from build123d import *

# Parameters (mm, degrees)
SKETCH1_W                                           = 150
SKETCH1_H                                           = 150
BOSS_EXTRUDE1_DEPTH                                 = 10
SKETCH2_R                                           = 45
SKETCH2_W                                           = 41
SKETCH2_H                                           = 21
BOSS_EXTRUDE2_DEPTH                                 = 35
SKETCH3_W                                           = 57
SKETCH3_H                                           = 21
CUT_EXTRUDE1_DEPTH                                  = 13
SKETCH5_W                                           = 57
SKETCH5_H                                           = 21
CUT_EXTRUDE3_DEPTH                                  = 29
RIB5_REACH                                          = 117.217
SKETCH6_WALL_W                                      = 276.297796834
SKETCH6_WALL_H                                      = 10
CIRPATTERN1_COUNT                                   = 4
CSK_FOR_M5_COUNTERSUNK_FLAT_HEAD_SCREW1_D           = 5.5
CSK_FOR_M5_COUNTERSUNK_FLAT_HEAD_SCREW1_CSINK_D     = 10.4
CSK_FOR_M5_COUNTERSUNK_FLAT_HEAD_SCREW1_CSINK_ANGLE = 90
SKETCH12_R                                          = 2.5
CUT_EXTRUDE4_DEPTH                                  = 10
CUT_EXTRUDE5_DEPTH                                  = 144.449259322
CUT_EXTRUDE5_DEPTH_BACK                             = 144.449259322
SKETCH13_W                                          = 5.5
SKETCH13_H                                          = 4


with BuildPart() as part:
    # Sketch1 → Boss-Extrude1 (new body)
    with BuildSketch(Plane(origin=(0, 0, 0), x_dir=(1, 0, 0), z_dir=(0, 1, 0))):
        Rectangle(SKETCH1_W, SKETCH1_H)
    extrude(amount=BOSS_EXTRUDE1_DEPTH)

    # Sketch2 → Boss-Extrude2 (add)
    with BuildSketch(Plane(origin=(0, 10, 0), x_dir=(1, 0, 0), z_dir=(0, 1, 0))):
        with Locations(Location((0, 0, 0), (0, 0, 270))):
            Circle(SKETCH2_R)
        with Locations((-10.2, 0)):
            Rectangle(SKETCH2_W, SKETCH2_H, mode=Mode.SUBTRACT)
    extrude(amount=BOSS_EXTRUDE2_DEPTH)

    # Sketch3 → Cut-Extrude1 (cut)
    with BuildSketch(Plane(origin=(0, 45, 0), x_dir=(1, 0, 0), z_dir=(0, 1, 0))):
        with Locations((-10.2, 0)):
            Rectangle(SKETCH3_W, SKETCH3_H)
    extrude(amount=-CUT_EXTRUDE1_DEPTH, mode=Mode.SUBTRACT)

    # Sketch5 → Cut-Extrude3 (cut)
    with BuildSketch(Plane.XZ):
        with Locations((-10.2, 0)):
            Rectangle(SKETCH5_W, SKETCH5_H)
    extrude(amount=-CUT_EXTRUDE3_DEPTH, mode=Mode.SUBTRACT)

    # Sketch6 wall → Rib5 (add, up to next)
    with BuildSketch(Plane(origin=(0, 26, -60), x_dir=(0, -0.72953720414, -0.683941128881), z_dir=(0, 0.683941128881, -0.72953720414)), mode=Mode.PRIVATE) as rib5_sk1:
        Rectangle(SKETCH6_WALL_W, SKETCH6_WALL_H)
    rib5_tool1 = extrude(rib5_sk1.sketch, amount=-RIB5_REACH, mode=Mode.PRIVATE) - part.part
    rib5 = rib5_tool1.solids().sort_by_distance((0, 26, -60))[0]
    add(rib5)

    # CirPattern1: Rib5 ×4 about axis
    cirpattern1_axis = Axis((0, 0, 0), (0, 1, 0))
    for i in range(1, CIRPATTERN1_COUNT):
        add(rib5.rotate(cirpattern1_axis, i * 360 / CIRPATTERN1_COUNT))

    # CSK for M5 Countersunk Flat Head Screw1 (through all)
    with Locations(Plane(origin=(0, 10, 0), x_dir=(1, 0, 0), z_dir=(0, 1, 0))):
        with Locations((55, -55), (-55, -55), (-55, 55), (55, 55)):
            CounterSinkHole(CSK_FOR_M5_COUNTERSUNK_FLAT_HEAD_SCREW1_D / 2, CSK_FOR_M5_COUNTERSUNK_FLAT_HEAD_SCREW1_CSINK_D / 2, counter_sink_angle=CSK_FOR_M5_COUNTERSUNK_FLAT_HEAD_SCREW1_CSINK_ANGLE)

    # Sketch12 → Cut-Extrude4 (cut)
    with BuildSketch(Plane(origin=(0, 32, 0), x_dir=(1, 0, 0), z_dir=(0, 1, 0))):
        with Locations(Location((-34.5, 5.25, 0), (0, 0, 270))):
            Circle(SKETCH12_R)
        with Locations(Location((-34.5, -4.75, 0), (0, 0, 270))):
            Circle(SKETCH12_R)
        with Locations(Location((14.5, 5.25, 0), (0, 0, 270))):
            Circle(SKETCH12_R)
        with Locations(Location((14.5, -5, 0), (0, 0, 270))):
            Circle(SKETCH12_R)
    extrude(amount=-CUT_EXTRUDE4_DEPTH, mode=Mode.SUBTRACT)

    # Sketch13 → Cut-Extrude5 (cut, two sides: drawn at the far end of the back side and taken through both)
    with BuildSketch(Plane(origin=(-38.7, 0, 0), x_dir=(0, 0, -1), z_dir=(1, 0, 0)).offset(-CUT_EXTRUDE5_DEPTH_BACK)):
        with Locations((0, 2)):
            Rectangle(SKETCH13_W, SKETCH13_H)
    extrude(amount=CUT_EXTRUDE5_DEPTH + CUT_EXTRUDE5_DEPTH_BACK, mode=Mode.SUBTRACT)


solid = part.part
Geometry check sheet. Reference: the model listing, model coordinates, mm. A direction names the side the tool comes from. Round coordinates to 2 decimals unless told otherwise and drop trailing zeros. Order: outer loops, then holes, each group sorted by start corner. A loop starts at its lowest first (then second) coordinate and runs counter-clockwise, first axis right, second up. Notation, with made-up numbers: M 67.5,-3 L 125.5,-3 A20 ccw 125.5,1 Z; hole C -6,-11.5 d4. An arc over 180 degrees is marked long. Answer in a Markdown table with one row per item. Add a question column.
Item 1: Draft check along X on faces 6 (the face through (-52.973, 3.722, -56.859)), 7 (the face through (5, 21, 53)), 8 (the face through (-35, 29, 0)), 9 (the face through (-48, 10, 47)). Enter one of: released by +X, released by -X, zero draft, split by the parting line, or undercut.
Item 2: Depth check by flat-ended pin: pin 1 Ø6.5 at (x, z) = (14.5, 5) entering from +Y; pin 2 Ø0.9 at (y, z) = (31, 4) entering from -X; pin 3 Ø9 at (y, z) = (19, -53) entering from +X. Enter the tip coordinate at first touch or a pass-through.
Item 3: Sectioned sample at D-D, the plane x = 55. Enter the section's corners in (y, z), plus the area to 3 significant figures.
Item 4: Sectioned sample at A-A, the plane x = 0. Enter the section's corners in (y, z), plus the area to 4 significant figures.
Item 5: Sectioned sample at B-B, the plane z = 0. Enter the section's corners in (x, y), plus the area to 3 significant figures.
Item 6: Set-up check for faces 1 (the face through (-17.235, 27.255, 41.569)), 2 (the face through (-5, 21, 53)), 3 (the face through (46, 4, 0)), 4 (the face through (53, 21, -5)), 5 (the face through (-1, 5, 75)): record each of +Z, -Z, +X, -X, +Y, -Y from which the full face is reachable in a straight line by a thin tool's end or side.
Item 7: Material ranges on L1, parallel to Z at x = -55, y = 6; L2, parallel to Z at x = 55, y = 2; L3, parallel to Z at x = -32, y = 9.5, recorded low to high. Write a range as [from, to].
Item 8: Sectioned sample at C-C, the plane y = 14. Enter the section's corners in (x, z).
Filled in:
| question | item | result |
|---|---|---|
| 1 | face 6 | undercut |
| 1 | face 7 | released by +X |
| 1 | face 8 | undercut |
| 1 | face 9 | zero draft |
| 2 | pin 1 | stops at y = 32 |
| 2 | pin 2 | stops at x = -55.73 |
| 2 | pin 3 | stops at x = 5 |
| 3 | outline | M 0,-75 L 10,-75 L 10,-60.2 L 7.55,-57.75 L 0,-57.75 Z; M 0,-52.25 L 7.55,-52.25 L 10,-49.8 L 10,-5 L 31.33,-5 L 31.33,5 L 10,5 L 10,49.8 L 7.55,52.25 L 0,52.25 L 0,2.75 L 4,2.75 L 4,-2.75 L 0,-2.75 Z; M 0,57.75 L 7.55,57.75 L 10,60.2 L 10,75 L 0,75 Z |
| 3 | area | 1,570 mm² |
| 4 | outline | M 0,-75 L 10,-75 L 42,-45 L 45,-45 L 45,-10.5 L 0,-10.5 Z; M 0,10.5 L 45,10.5 L 45,45 L 42,45 L 10,75 L 0,75 Z |
| 4 | area | 4,665 mm² |
| 5 | outline | M -75,4 L -38.7,4 L -38.7,29 L -30.7,29 L -30.7,32 L -38.7,32 L -38.7,45 L -45,45 L -45,42 L -75,10 Z; M 10.3,29 L 18.3,29 L 18.3,4 L 75,4 L 75,10 L 45,42 L 45,45 L 18.3,45 L 18.3,32 L 10.3,32 Z |
| 5 | area | 2,720 mm² |
| 6 | face 1 | +Y |
| 6 | face 2 | +Z, -X, +Y |
| 6 | face 3 | +X, -X, -Y |
| 6 | face 4 | -Z, +X, +Y |
| 6 | face 5 | +Z, +X, -X, +Y, -Y |
| 7 | L1 | z = [-75, -57.75], [-52.25, 52.25], [57.75, 75] |
| 7 | L2 | z = [-75, -57.75], [-52.25, -2.75], [2.75, 52.25], [57.75, 75] |
| 7 | L3 | z = [-75, -10.5], [10.5, 75] |
| 8 | outline | M -71.25,-5 L -44.72,-5 A45 ccw -5,-44.72 L -5,-71.25 L 5,-71.25 L 5,-44.72 A45 ccw 44.72,-5 L 71.25,-5 L 71.25,5 L 44.72,5 A45 ccw 5,44.72 L 5,71.25 L -5,71.25 L -5,44.72 A45 ccw -44.72,5 L -71.25,5 Z; hole M -38.7,-10.5 L 18.3,-10.5 L 18.3,10.5 L -38.7,10.5 Z |
